from build123d import *

# Parameters (mm, degrees)
SKETCH1_W               = 51.3
SKETCH1_H               = 18.5
BOSS_EXTRUDE1_DEPTH     = 12.4
SKETCH2_R               = 3.2
CUT_EXTRUDE1_DEPTH      = 34.969581982
SKETCH3_R               = 2.45
CUT_EXTRUDE2_DEPTH      = 30.95404814
CHAMFER1_SIZE           = 1
SKETCH4_R               = 3.45
BOSS_EXTRUDE2_DEPTH     = 3
MIRROR3_COPY_1_SKETCH_R = 3.45
MIRROR3_COPY_1_DEPTH    = 3


with BuildPart() as part:
    # Sketch1 → Boss-Extrude1 (new body)
    with BuildSketch(Plane(origin=(0, 0, 0), x_dir=(1, 0, 0), z_dir=(0, 1, 0))):
        Rectangle(SKETCH1_W, SKETCH1_H)
    extrude(amount=BOSS_EXTRUDE1_DEPTH)

    # Sketch2 → Cut-Extrude1 (cut, through all)
    with BuildSketch(Plane.XY.offset(9.25)):
        with Locations((4.45, 6.2)):
            Circle(SKETCH2_R)
        with Locations((12.75, 6.2)):
            Circle(SKETCH2_R)
    cut_extrude1 = extrude(amount=-CUT_EXTRUDE1_DEPTH, mode=Mode.SUBTRACT)

    # Sketch3 → Cut-Extrude2 (cut, through all)
    with BuildSketch(Plane(origin=(0, 12.4, 0), x_dir=(1, 0, 0), z_dir=(0, 1, 0))):
        with Locations(Location((20.6, 0, 0), (0, 0, 270))):
            Circle(SKETCH3_R)
    cut_extrude2 = extrude(amount=-CUT_EXTRUDE2_DEPTH, mode=Mode.SUBTRACT)

    # Mirror1: Cut-Extrude1, Cut-Extrude2 across plane
    add(cut_extrude1.mirror(Plane(origin=(0, 0, 0), x_dir=(0, 0, 1), z_dir=(1, 0, 0))), mode=Mode.SUBTRACT)
    add(cut_extrude2.mirror(Plane(origin=(0, 0, 0), x_dir=(0, 0, 1), z_dir=(1, 0, 0))), mode=Mode.SUBTRACT)

    # Chamfer1
    chamfer1_edges = [part.edges().sort_by_distance(p)[0] for p in [
        (20.6, 12.4, -2.45),
        (-20.6, 12.4, -2.45),
    ]]
    chamfer(chamfer1_edges, length=CHAMFER1_SIZE)

    # Sketch4 → Boss-Extrude2 (add)
    with BuildSketch(Plane(origin=(0, 12.4, 0), x_dir=(1, 0, 0), z_dir=(0, 1, 0))):
        with Locations(Location((4.45, -5.25, 0), (0, 0, 270))):
            Circle(SKETCH4_R)
        with Locations(Location((12.75, -5.25, 0), (0, 0, 270))):
            Circle(SKETCH4_R)
    boss_extrude2 = extrude(amount=BOSS_EXTRUDE2_DEPTH)

    # Mirror2: Boss-Extrude2 across plane
    add(boss_extrude2.mirror(Plane.XY))

    # Mirror3: Boss-Extrude2 across plane
    add(boss_extrude2.mirror(Plane(origin=(0, 0, 0), x_dir=(0, 0, 1), z_dir=(1, 0, 0))))

    # Mirror3 copy 1 sketch → Mirror3 copy 1 (add)
    with BuildSketch(Plane(origin=(0, 12.4, 0), x_dir=(-1, 0, 0), z_dir=(0, 1, 0))):
        with Locations(Location((4.45, -5.25, 0), (0, 0, 270))):
            Circle(MIRROR3_COPY_1_SKETCH_R)
        with Locations(Location((12.75, -5.25, 0), (0, 0, 270))):
            Circle(MIRROR3_COPY_1_SKETCH_R)
    extrude(amount=MIRROR3_COPY_1_DEPTH)


solid = part.part
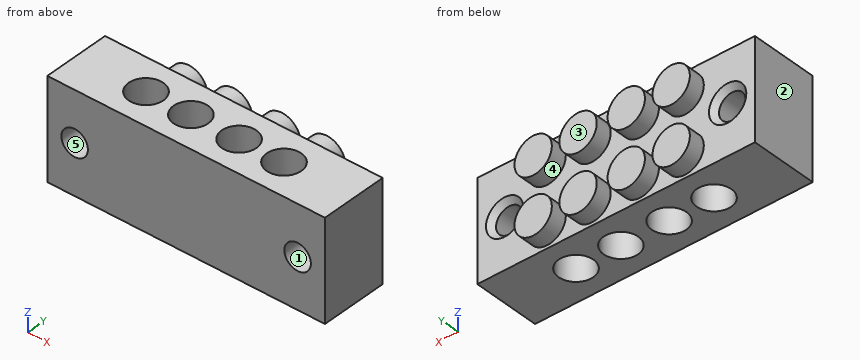
Verification items for the finished model (mm, model axes). Face numbers are marked on the shaded views. A direction names the side the tool comes from. Give positions to 0.01 mm unless a question says otherwise; leave off trailing zeros. Order: outer loops, then holes, each group sorted by start corner. A loop starts at its lowest first (then second) coordinate and runs counter-clockwise, first axis right, second up. Notation, with made-up numbers: M -1.5,38.5 L 54.5,38.5 A22 ccw 54.5,47.5 Z; hole C -6,14.25 d3. An arc over 180 degrees is marked long. Use one line per item in the form item = value. Start each with the question number.
Q1. Mould release check, pull along X, two halves, no side actions. Record for the marked faces 1, 2 and 3: +X half, -X half, draft (parallel to the pull), parting line (faces both ways), or undercut.
Q2. Go/stop test with a flat-tipped pin: pin 1 Ø6.5 at (x, z) = (-20.6, 0) entering from +Y. Record where the tip stops, or that it passes through.
Q3. Access from +Z, -Z, +X, -X, +Y, -Y to the whole of each face (thin tool, end or side, straight path). Record for the marked faces 4 and 5.
Q4. Section check C-C (z = -5.25). Enter the section's corners in (x, y), then the cut area to 3 significant figures.
Q5. Section check B-B (y = 13.25). Enter the section's corners in (x, z), then the cut area to 3 significant figures.
Q6. Section check D-D (x = 20.6). Enter the section's corners in (y, z).
Q7. Scan lines: line 1 along X through (y, z) = (13.5, -5); line 2 along X through (y, z) = (1.25, 0); line 3 along Y through (x, z) = (12.75, -4.5). Record each from-to range of solid material in increasing order. Write a range as [from, to].
Q8. Section check A-A (y = 6.2). Enter the section's corners in (x, z).
Evaluation:
q1.face_1 = undercut
q1.face_2 = -X half
q1.face_3 = draft
q2.pin_1 = 12.2
q3.face_4 = +Y
q3.face_5 = +Y, -Y
q4.outline = M -25.65,0 L 25.65,0 L 25.65,12.4 L 16.2,12.4 L 16.2,15.4 L 9.3,15.4 L 9.3,12.4 L 7.9,12.4 L 7.9,15.4 L 1,15.4 L 1,12.4 L -1,12.4 L -1,15.4 L -7.9,15.4 L -7.9,12.4 L -9.3,12.4 L -9.3,15.4 L -16.2,15.4 L -16.2,12.4 L -25.65,12.4 Z; hole C -12.75,6.2 d6.4; hole C -4.45,6.2 d6.4; hole C 4.45,6.2 d6.4; hole C 12.75,6.2 d6.4
q4.area = 590 mm2
q5.outline = C -12.75,-5.25 d6.9; C -12.75,5.25 d6.9; C -4.45,-5.25 d6.9; C -4.45,5.25 d6.9; C 4.45,-5.25 d6.9; C 4.45,5.25 d6.9; C 12.75,-5.25 d6.9; C 12.75,5.25 d6.9
q5.area = 299 mm2
q6.outline = M 0,-9.25 L 12.4,-9.25 L 12.4,-3.45 L 11.4,-2.45 L 0,-2.45 Z; M 0,2.45 L 11.4,2.45 L 12.4,3.45 L 12.4,9.25 L 0,9.25 Z
q7.line_1 = [-16.19, -9.31], [-7.89, -1.01], [1.01, 7.89], [9.31, 16.19]
q7.line_2 = [-25.65, -23.05], [-18.15, 18.15], [23.05, 25.65]
q7.line_3 = [0, 3], [9.4, 15.4]
q8.outline = M -25.65,-9.25 L -15.95,-9.25 L -15.95,9.25 L -25.65,9.25 Z; M -9.55,-9.25 L -7.65,-9.25 L -7.65,9.25 L -9.55,9.25 Z; M -1.25,-9.25 L 1.25,-9.25 L 1.25,9.25 L -1.25,9.25 Z; M 7.65,-9.25 L 9.55,-9.25 L 9.55,9.25 L 7.65,9.25 Z; M 15.95,-9.25 L 25.65,-9.25 L 25.65,9.25 L 15.95,9.25 Z; hole C -20.6,0 d4.9; hole C 20.6,0 d4.9
